Read the model definition and answer for the solid it produces. Units are mm, in the model's axes. A direction names the side the tool comes from. Round coordinates to 2 decimals unless told otherwise and drop trailing zeros. Write each loop counter-clockwise with the first axis right and the second up, starting at its lowest first coordinate (ties: lowest second). Pieces come first, ordered by that corner, then holes. Notation, with made-up numbers: (14, 46.25) -> (72, 46.25) arc R21 cw to (72, 72.25) -> close; hole circle Ø10 at (81.5, 19.5). An arc over 180 degrees is marked (long way). Return JSON: item names as keys, results as strings. Group by question number.
(1) For faces 4 (the flat face through (-18, -16, 51)), 5 (the flat face through (18, -3, 31)), 6 (the flat face through (48, -29, 46)), determine the directions among +Z, -Z, +X, -X, +Y, -Y from which every point of the face is accessible in a straight line to the end or side of a thin tool.
(2) Given pin 1 (1.1 mm diameter, centred on x = -7.5, z = 34.5, fed in from -Y); pin 2 (2 mm diameter, centred on x = 24.5, y = 18, fed in from +Z); pin 3 (10 mm diameter, centred on x = 40, z = 36.5, fed in from +Y); pin 4 (3 mm diameter, centred on x = -13, z = 9, fed in from +Y), each flat-ended and moving along its own axis, determine where each tip first touches the part or whether it passes through.
(3) The mould has two halves that part along Z. Classify faces 1 (the flat face through (39, -16, 51)), 2 (the flat face through (3.9, 23, 34.4)), 3 (the flat face through (18, 22, 33)): released by +Z, released by -Z, zero draft, split by the parting line, or undercut.
(4) A cutting plane is placed at B-B on z = 15.5. Give the vertices of the cut face in (x, y).
(5) Straight lines are drawn through the part: line 1 (Z direction, x = 22.5, y = -22); line 2 (X direction, y = 8, z = 37.5); line 3 (Z direction, x = 34.5, y = 0.5). For each, find the intervals that lie inside material, in ascending order.
(6) A cutting plane is placed at A-A on y = -8. State how many separate pieces and enclosed holes the cut face has, then the cut area to 3 significant figures.
```python
from build123d import *

# Parameters (mm, degrees)
SKETCH_W        = 100
SKETCH_H        = 60
PAD_DEPTH       = 30
SKETCH001_W     = 98
SKETCH001_H     = 28
POCKET_DEPTH    = 58
SKETCH002_W     = 96
SKETCH002_H     = 3
POCKET001_DEPTH = 60.001
SKETCH003_W     = 96
SKETCH003_H     = 4
POCKET002_DEPTH = 60.001
SKETCH007_W     = 96
SKETCH007_H     = 4
POCKET003_DEPTH = 60.001
SKETCH008_W     = 96
SKETCH008_H     = 4
POCKET004_DEPTH = 60.001
SKETCH009_W     = 96
SKETCH009_H     = 3
POCKET005_DEPTH = 60.001
POCKET006_DEPTH = 2
PAD001_DEPTH    = 100
SKETCH012_W     = 20
SKETCH012_H     = 20
SKETCH012_W_2   = 14
POCKET007_DEPTH = 50
SKETCH013_W     = 96
SKETCH013_H     = 4
POCKET008_DEPTH = 2
SKETCH014_W     = 96
SKETCH014_H     = 4
POCKET009_DEPTH = 2
SKETCH015_W     = 96
SKETCH015_H     = 4
POCKET010_DEPTH = 2
FILLET_R        = 1
CHAMFER_SIZE    = 0.5
CHAMFER001_SIZE = 0.2
CHAMFER002_SIZE = 0.2
CHAMFER003_SIZE = 0.2
FILLET001_R     = 0.5
CHAMFER004_SIZE = 0.5


with BuildPart() as part:
    # Sketch → Pad (new body)
    with BuildSketch(Plane.XY):
        Rectangle(SKETCH_W, SKETCH_H)
    extrude(amount=PAD_DEPTH)

    # Sketch001 → Pocket (cut)
    with BuildSketch(Plane.XZ.offset(-30)):
        with Locations((0, 15)):
            Rectangle(SKETCH001_W, SKETCH001_H)
    extrude(amount=POCKET_DEPTH, mode=Mode.SUBTRACT)

    # Sketch002 → Pocket001 (cut, through all)
    with BuildSketch(Plane.XZ.offset(30)):
        with Locations((0, 26.5)):
            Rectangle(SKETCH002_W, SKETCH002_H)
    extrude(amount=-POCKET001_DEPTH, mode=Mode.SUBTRACT)

    # Sketch003 → Pocket002 (cut, through all)
    with BuildSketch(Plane.XZ.offset(30)):
        with Locations((0, 21)):
            Rectangle(SKETCH003_W, SKETCH003_H)
    extrude(amount=-POCKET002_DEPTH, mode=Mode.SUBTRACT)

    # Sketch007 → Pocket003 (cut, through all)
    with BuildSketch(Plane.XZ.offset(30)):
        with Locations((0, 15)):
            Rectangle(SKETCH007_W, SKETCH007_H)
    extrude(amount=-POCKET003_DEPTH, mode=Mode.SUBTRACT)

    # Sketch008 → Pocket004 (cut, through all)
    with BuildSketch(Plane.XZ.offset(30)):
        with Locations((0, 9)):
            Rectangle(SKETCH008_W, SKETCH008_H)
    extrude(amount=-POCKET004_DEPTH, mode=Mode.SUBTRACT)

    # Sketch009 → Pocket005 (cut, through all)
    with BuildSketch(Plane.XZ.offset(30)):
        with Locations((0, 3.5)):
            Rectangle(SKETCH009_W, SKETCH009_H)
    extrude(amount=-POCKET005_DEPTH, mode=Mode.SUBTRACT)

    # Sketch010 → Pocket006 (cut)
    with BuildSketch(Plane.XY):
        with BuildLine():
            Line((-3.5, 21.062178), (3.5, 21.062178))
            Line((3.5, 21.062178), (3.5, 11.062178))
            ThreePointArc((-3.5, 11.062178), (0, -2), (3.5, 11.062178))
            Line((-3.5, 11.062178), (-3.5, 21.062178))
        make_face()
    extrude(amount=POCKET006_DEPTH, mode=Mode.SUBTRACT)

    # Sketch011 → Pad001 (join)
    with BuildSketch(Plane.YZ.offset(50)):
        Polygon((-30, 52), (-30, 30), (30, 30), (-5, 52), align=None)
    extrude(amount=-PAD001_DEPTH)

    # Sketch012 → Pocket007 (cut)
    with BuildSketch(Plane.XZ.offset(28)):
        with Locations((39, 41)):
            Rectangle(SKETCH012_W, SKETCH012_H)
        with Locations((18, 41)):
            Rectangle(SKETCH012_W, SKETCH012_H)
        with Locations((-39, 41)):
            Rectangle(SKETCH012_W, SKETCH012_H)
        with Locations((-18, 41)):
            Rectangle(SKETCH012_W, SKETCH012_H)
        with Locations((0, 41)):
            Rectangle(SKETCH012_W_2, SKETCH012_H)
    extrude(amount=-POCKET007_DEPTH, mode=Mode.SUBTRACT)

    # Sketch013 → Pocket008 (cut)
    with BuildSketch(Plane.XZ.offset(30)):
        with Locations((0, 34)):
            Rectangle(SKETCH013_W, SKETCH013_H)
    extrude(amount=-POCKET008_DEPTH, mode=Mode.SUBTRACT)

    # Sketch014 → Pocket009 (cut)
    with BuildSketch(Plane.XZ.offset(30)):
        with Locations((0, 40)):
            Rectangle(SKETCH014_W, SKETCH014_H)
    extrude(amount=-POCKET009_DEPTH, mode=Mode.SUBTRACT)

    # Sketch015 → Pocket010 (cut)
    with BuildSketch(Plane.XZ.offset(30)):
        with Locations((0, 46)):
            Rectangle(SKETCH015_W, SKETCH015_H)
    extrude(amount=-POCKET010_DEPTH, mode=Mode.SUBTRACT)

    # Fillet
    fillet_edges = [part.edges().sort_by_distance(p)[0] for p in [
        (-50, -17.5, 52),
        (50, -17.5, 52),
        (50, 0, 0),
        (50, -30, 26),
        (0, -30, 52),
        (0, -30, 0),
        (-50, -30, 26),
        (-50, 0, 0),
    ]]
    fillet(fillet_edges, radius=FILLET_R)

    # Chamfer
    chamfer_edges = [part.edges().sort_by_distance(p)[0] for p in [
        (50, 13.295455, 40.5),
        (-50, 13.295455, 40.5),
    ]]
    chamfer(chamfer_edges, length=CHAMFER_SIZE)

    # Chamfer001
    chamfer001_edges = [part.edges().sort_by_distance(p)[0] for p in [
        (-29, 9.295455, 43.014286),
        (-28, 9.295455, 43.014286),
    ]]
    chamfer(chamfer001_edges, length=CHAMFER001_SIZE)

    # Chamfer002
    chamfer002_edges = [part.edges().sort_by_distance(p)[0] for p in [
        (7, 9.295455, 43.014286),
        (8, 9.295455, 43.014286),
        (-8, 9.295455, 43.014286),
        (-7, 9.295455, 43.014286),
        (28, 9.295455, 43.014286),
        (29, 9.295455, 43.014286),
    ]]
    chamfer(chamfer002_edges, length=CHAMFER002_SIZE)

    # Chamfer003
    chamfer003_edges = [part.edges().sort_by_distance(p)[0] for p in [
        (49, 9.295455, 43.014286),
        (-49, 9.295455, 43.014286),
    ]]
    chamfer(chamfer003_edges, length=CHAMFER003_SIZE)

    # Fillet001
    fillet001_edges = [part.edges().sort_by_distance(p)[0] for p in [
        (49, 30, 15),
        (0, 30, 29),
        (0, 30, 1),
        (-49, 30, 15),
    ]]
    fillet(fillet001_edges, radius=FILLET001_R)

    # Chamfer004
    chamfer004_edges = [part.edges().sort_by_distance(p)[0] for p in [
        (0, -2, 0),
        (3.5, 16.062178, 0),
        (-3.5, 16.062178, 0),
    ]]
    chamfer(chamfer004_edges, length=CHAMFER004_SIZE)


solid = part.part
```
Checks:
{
 "1": {"face 4": "+Y", "face 5": "none", "face 6": "+Y, -Y"},
 "2": {"pin 1": "stops at y = -28", "pin 2": "stops at z = 31", "pin 3": "stops at y = 27.61", "pin 4": "passes through"},
 "3": {"face 1": "undercut", "face 2": "released by +Z", "face 3": "zero draft"},
 "4": {"outline": "(-50, -29) arc R1 ccw to (-49, -30) -> (-48, -30) -> (-48, -28) -> (-49, -28) -> (-49, 29.5) arc R0.5 ccw to (-49.5, 30) -> (-50, 30) -> close; (48, -30) -> (49, -30) arc R1 ccw to (50, -29) -> (50, 30) -> (49.5, 30) arc R0.5 ccw to (49, 29.5) -> (49, -28) -> (48, -28) -> close"},
 "5": {"line 1": "z = 0 to 1, 29 to 31, 51 to 52", "line 2": "x = -50 to -49, -29 to -28, -8 to -7, 7 to 8, 28 to 29, 49 to 50", "line 3": "z = 0 to 1, 29 to 31"},
 "6": {"separate pieces": "1", "enclosed holes": "6", "area": "575 mm^2"}
}
